from build123d import *

# Parameters (mm, degrees)
SKETCH1_W           = 30
SKETCH1_H           = 47.5
BOSS_EXTRUDE1_DEPTH = 6
BOSS_EXTRUDE2_DEPTH = 30
BOSS_EXTRUDE3_DEPTH = 3
BOSS_EXTRUDE4_DEPTH = 12.5
SKETCH5_R           = 2.25
CUT_EXTRUDE1_DEPTH  = 49.106652347
SKETCH8_W           = 20
SKETCH8_H           = 15
CUT_EXTRUDE4_DEPTH  = 58.456505289
SKETCH9_R           = 2.25
CUT_EXTRUDE5_DEPTH  = 44.200115741
CUT_EXTRUDE6_DEPTH  = 5
CHAMFER1_SIZE       = 4
CUT_EXTRUDE7_DEPTH  = 44.200115741


with BuildPart() as part:
    # Sketch1 → Boss-Extrude1 (new body)
    with BuildSketch(Plane(origin=(0, 0, 0), x_dir=(0, 0, -1), z_dir=(1, 0, 0))):
        with Locations((0, -15.75)):
            Rectangle(SKETCH1_W, SKETCH1_H)
    extrude(amount=BOSS_EXTRUDE1_DEPTH)

    # Sketch2 → Boss-Extrude2 (add)
    with BuildSketch(Plane.XY.offset(15)):
        with BuildLine():
            Line((6, -39.5), (16.5, -39.5))
            Line((16.5, -39.5), (16.5, -32))
            ThreePointArc((16.5, -32), (11.196699141, -29.803300859), (9, -24.5))
            Line((9, -24.5), (9, -9.5))
            Line((9, -9.5), (6, -9.5))
            Line((6, -9.5), (6, -39.5))
        make_face()
    extrude(amount=-BOSS_EXTRUDE2_DEPTH)

    # Sketch3 → Boss-Extrude3 (add)
    with BuildSketch(Plane.XY.offset(15)):
        with BuildLine():
            Line((16.5, -29.5), (16.5, -32))
            ThreePointArc((16.5, -32), (11.196699141, -29.803300859), (9, -24.5))
            Line((9, -24.5), (11.5, -24.5))
            ThreePointArc((11.5, -24.5), (12.964466094, -28.035533906), (16.5, -29.5))
        make_face()
    boss_extrude3 = extrude(amount=-BOSS_EXTRUDE3_DEPTH)

    # Mirror1: Boss-Extrude3 across plane
    add(boss_extrude3.mirror(Plane.XY))

    # Sketch4 → Boss-Extrude4 (add)
    with BuildSketch(Plane(origin=(16.5, 0, 0), x_dir=(0, 0, -1), z_dir=(1, 0, 0))):
        Polygon((-12, -32), (12, -32), (12, -29.5), (15, -29.5), (15, -39.5), (-15, -39.5), (-15, -29.5), (-12, -29.5), align=None)
    extrude(amount=BOSS_EXTRUDE4_DEPTH)

    # Sketch5 → Cut-Extrude1 (cut, through all)
    with BuildSketch(Plane(origin=(6, 0, 0), x_dir=(0, 0, -1), z_dir=(1, 0, 0))):
        with Locations((-12, 0)):
            Circle(SKETCH5_R)
        with Locations((12, 0)):
            Circle(SKETCH5_R)
    extrude(amount=-CUT_EXTRUDE1_DEPTH, mode=Mode.SUBTRACT)

    # Sketch8 → Cut-Extrude4 (cut, through all)
    with BuildSketch(Plane.XY.offset(15)):
        with Locations((19, -32)):
            Rectangle(SKETCH8_W, SKETCH8_H)
    extrude(amount=-CUT_EXTRUDE4_DEPTH, mode=Mode.SUBTRACT)

    # Sketch9 → Cut-Extrude5 (cut, through all)
    with BuildSketch(Plane(origin=(9, 0, 0), x_dir=(0, 0, -1), z_dir=(1, 0, 0))):
        with Locations((-9, -14.5)):
            Circle(SKETCH9_R)
        with Locations((9, -14.5)):
            Circle(SKETCH9_R)
        with Locations((9, -34.5)):
            Circle(SKETCH9_R)
        with Locations((-9, -34.5)):
            Circle(SKETCH9_R)
    extrude(amount=-CUT_EXTRUDE5_DEPTH, mode=Mode.SUBTRACT)

    # Sketch10 → Cut-Extrude6 (cut)
    with BuildSketch(Plane.ZY):
        Polygon((-13.041451884, -14.5), (-11.020725942, -18), (-6.979274058, -18), (-4.958548116, -14.5), (-6.979274058, -11), (-11.020725942, -11), align=None)
        Polygon((4.958548116, -14.5), (6.979274058, -18), (11.020725942, -18), (13.041451884, -14.5), (11.020725942, -11), (6.979274058, -11), align=None)
        Polygon((4.958548116, -34.5), (6.979274058, -38), (11.020725942, -38), (13.041451884, -34.5), (11.020725942, -31), (6.979274058, -31), align=None)
        Polygon((-13.041451884, -34.5), (-11.020725942, -38), (-6.979274058, -38), (-4.958548116, -34.5), (-6.979274058, -31), (-11.020725942, -31), align=None)
    extrude(amount=-CUT_EXTRUDE6_DEPTH, mode=Mode.SUBTRACT)

    # Chamfer1
    chamfer1_edges = [part.edges().sort_by_distance(p)[0] for p in [
        (3, 8, -15),
        (3, 8, 15),
    ]]
    chamfer(chamfer1_edges, length=CHAMFER1_SIZE)

    # Sketch12 → Cut-Extrude7 (cut, through all)
    with BuildSketch(Plane(origin=(9, 0, 0), x_dir=(0, 0, -1), z_dir=(1, 0, 0))):
        Polygon((-2.25, -39.5), (2.25, -39.5), (2.25, -35.5), (3.5, -35.5), (3.5, -30.5), (2.25, -30.5), (2.25, -26.5), (-2.25, -26.5), (-2.25, -30.5), (-3.5, -30.5), (-3.5, -35.5), (-2.25, -35.5), align=None)
    extrude(amount=-CUT_EXTRUDE7_DEPTH, mode=Mode.SUBTRACT)


solid = part.part
Input: part model. Units: mm. Frame: model coordinates. A direction names the side the tool comes from. Round coordinates to 2 decimals unless told otherwise and drop trailing zeros. Order: outer loops, then holes, each group sorted by start corner. A loop starts at its lowest first (then second) coordinate and runs counter-clockwise, first axis right, second up.
1. Cut plane B-B, the plane x = 7.25. Output: boundary loops of the cut face in (y, z).
The answers:
outline: (-39.5, -15) - (-9.5, -15) - (-9.5, 15) - (-39.5, 15) - (-39.5, 2.25) - (-35.5, 2.25) - (-35.5, 3.5) - (-30.5, 3.5) - (-30.5, 2.25) - (-26.5, 2.25) - (-26.5, -2.25) - (-30.5, -2.25) - (-30.5, -3.5) - (-35.5, -3.5) - (-35.5, -2.25) - (-39.5, -2.25) - close; hole circle Ø4.5 at (-34.5, -9); hole circle Ø4.5 at (-34.5, 9); hole circle Ø4.5 at (-14.5, -9); hole circle Ø4.5 at (-14.5, 9)
2. Cut plane D-D, the plane z = -9. Output: boundary loops of the cut face in (x, y).
The answers:
outline: (0, -39.5) - (9, -39.5) - (9, -36.75) - (5, -36.75) - (5, -38) - (0, -38) - close; (0, -31) - (5, -31) - (5, -32.25) - (9, -32.25) - (9, -16.75) - (5, -16.75) - (5, -18) - (0, -18) - close; (0, -11) - (5, -11) - (5, -12.25) - (9, -12.25) - (9, -9.5) - (6, -9.5) - (6, 8) - (0, 8) - close
3. Material intervals for line 1 (Y direction, x = 7, z = 9); line 2 (Z direction, x = 6.25, y = -37); line 3 (Y direction, x = 4.75, z = -6), sorted ascending.
The answers:
line 1: y = -39.5 to -36.75, -32.25 to -16.75, -12.25 to -9.5
line 2: z = -15 to -2.25, 2.25 to 15
line 3: y = -39.5 to -36.3, -32.7 to -16.3, -12.7 to 8
4. Set-up query: faces 3 (the face through (5, -37, 2.25)), 4 (the face through (4, -17, -15)), 5 (the face through (5, -13, 11)), 6 (the face through (5, -33, -3.5)). Return all of +Z, -Z, +X, -X, +Y, -Y with unobstructed straight access to the full face (end or side cutting, diameter ignored); none if empty.
The answers:
face 3: +X, -X, -Y
face 4: -Z, +X, -X, +Y, -Y
face 5: -X
face 6: +X, -X
5. Cut plane C-C, the plane y = 0. Output: boundary loops of the cut face in (x, z), then the cut area to 3 significant figures.
The answers:
outline: (0, -15) - (6, -15) - (6, -14.25) - (0, -14.25) - close; (0, -9.75) - (6, -9.75) - (6, 9.75) - (0, 9.75) - close; (0, 14.25) - (6, 14.25) - (6, 15) - (0, 15) - close
area: 126 mm2
6. Cut plane A-A, the plane z = -3. Output: boundary loops of the cut face in (x, y), then the cut area to 3 significant figures.
The answers:
outline: (0, -39.5) - (9, -39.5) - (9, -35.5) - (0, -35.5) - close; (0, -30.5) - (9, -30.5) - (9, -9.5) - (6, -9.5) - (6, 8) - (0, 8) - close
area: 330 mm2
7. Pin query (flat end, axial travel): P1, Ø5, axis at x = 2.5, z = -1, coming from the -Y side; P2, Ø5, axis at y = -14.5, z = -9, coming from the -X side; P3, Ø2, axis at y = -14, z = -8, coming from the -X side; P4, Ø1.5, axis at x = 7, z = 0, coming from the +Y side. Return the tip coordinate at first contact, or that it passes through.
The answers:
P1: stops at y = -39.5
P2: stops at x = 5
P3: passes through
P4: stops at y = -9.5
8. Mould query, pull axis Z, two halves, no side actions, for faces 1 (the face through (3, 6, -13)), 2 (the face through (2.5, -36.3, 12)). Classes: released by +Z, released by -Z, zero draft, split by the parting line, or undercut.
The answers:
face 1: released by -Z
face 2: undercut
